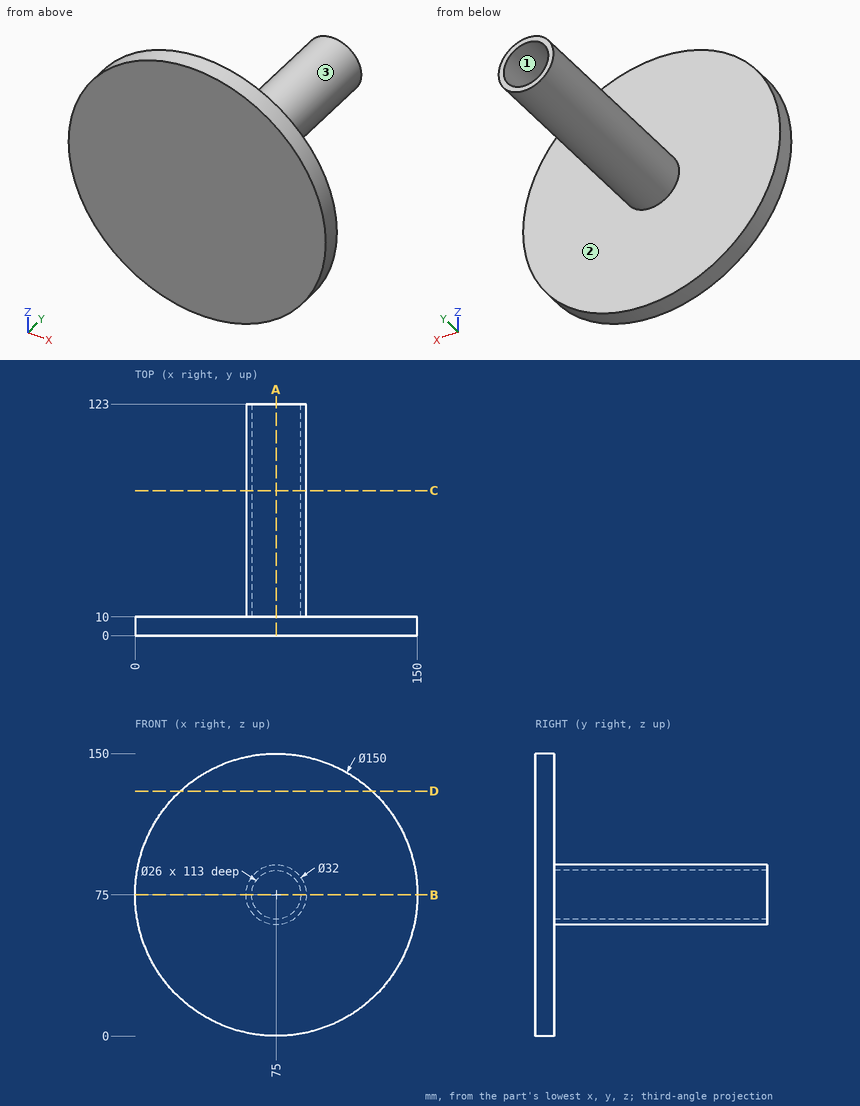
Geometry: see drawing. Coordinates: mm, zero at the bounding-box minimum. Give positions to 0.01 mm unless a question says otherwise; leave off trailing zeros. Loops run counter-clockwise (first coordinate to the right, second up) from the corner with the lowest first, then second, coordinate; pieces in that order, holes last. Notation, with made-up numbers: (27, 27) -> (66, 27) arc R19 ccw to (66, 50) -> close; hole circle Ø10 at (69, -27.75). An arc over 180 degrees is marked (long way). Put each result on its own line as item: value.
1. Cut plane A-A (x = 75). Return the cut outline in (y, z).
Taken from the geometry:
outline: (0, 0) -> (10, 0) -> (10, 59) -> (123, 59) -> (123, 62) -> (10, 62) -> (10, 88) -> (123, 88) -> (123, 91) -> (10, 91) -> (10, 150) -> (0, 150) -> close
2. Pin query (flat end, axial travel): P1, Ø1, axis at x = 64, y = 32.5, coming from the +Z side; P2, Ø2, axis at x = 82, y = 16, coming from the +Z side; P3, Ø1.5, axis at y = 64.5, z = 81.5, coming from the +X side; P4, Ø21, axis at x = 80, z = 79.5, coming from the +Y side. Return the tip coordinate at first contact, or that it passes through.
Taken from the geometry:
P1: stops at z = 87.07
P2: stops at z = 89.83
P3: stops at x = 89.93
P4: stops at y = 123
3. Ray query, line 1 along Z through (x, y) = (75, 78); line 2 along Y through (x, z) = (73, 81.5). Return the intervals inside material, ascending. Write a range as [from, to].
Taken from the geometry:
line 1: z = [59, 62], [88, 91]
line 2: y = [0, 10]
4. Cut plane B-B (z = 75). Return the cut outline in (x, y).
Taken from the geometry:
outline: (0, 0) -> (150, 0) -> (150, 10) -> (91, 10) -> (91, 123) -> (88, 123) -> (88, 10) -> (62, 10) -> (62, 123) -> (59, 123) -> (59, 10) -> (0, 10) -> close
5. Cut plane C-C (y = 77). Return the cut outline in (x, z), plus the area to 3 significant figures.
Taken from the geometry:
outline: circle Ø32 at (75, 75); hole circle Ø26 at (75, 75)
area: 273 mm2
6. Pull-direction query (Z, two-part tool) for the marked faces 1, 2 and 3; classes: released by +Z, released by -Z, zero draft, split by the parting line, or undercut.
Taken from the geometry:
face 1: undercut
face 2: zero draft
face 3: split by the parting line
7. Cut plane D-D (z = 130). Return the cut outline in (x, y), plus the area to 3 significant figures.
Taken from the geometry:
outline: (24.01, 0) -> (125.99, 0) -> (125.99, 10) -> (24.01, 10) -> close
area: 1,020 mm2
